```python
from build123d import *

# Parameters (mm, degrees)
SKETCH1_W           = 24.5
SKETCH1_H           = 20.5
BOSS_EXTRUDE1_DEPTH = 4.5
SKETCH2_W           = 0.25
SKETCH2_H           = 0.7
BOSS_EXTRUDE2_DEPTH = 3.5


with BuildPart() as part:
    # Sketch1 → Boss-Extrude1 (new body)
    with BuildSketch(Plane(origin=(0, 0, 0), x_dir=(0, 0, -1), z_dir=(1, 0, 0))):
        Rectangle(SKETCH1_W, SKETCH1_H)
    extrude(amount=BOSS_EXTRUDE1_DEPTH)

    # Sketch2 → Boss-Extrude2 (add)
    with BuildSketch(Plane.XZ.offset(10.25)):
        with Locations((1.2, 7.62)):
            Rectangle(SKETCH2_W, SKETCH2_H)
        with Locations((1.2, 10.16)):
            Rectangle(SKETCH2_W, SKETCH2_H)
        with Locations((1.2, -2.54)):
            Rectangle(SKETCH2_W, SKETCH2_H)
        with Locations((1.2, -10.16)):
            Rectangle(SKETCH2_W, SKETCH2_H)
    extrude(amount=BOSS_EXTRUDE2_DEPTH)


solid = part.part
```
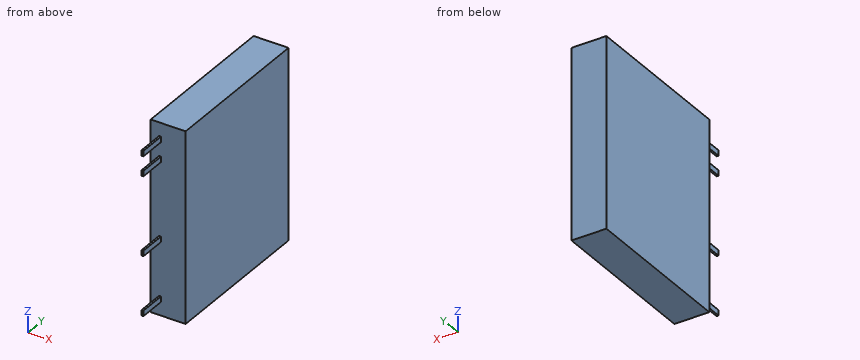
Source: CAD feature listing. Evaluate the final solid. Frame: model axes, mm. Give positions to 0.01 mm unless a question says otherwise; leave off trailing zeros. Write each loop counter-clockwise with the first axis right and the second up, starting at its lowest first coordinate (ties: lowest second). Pieces come first, ordered by that corner, then holes.
1. Section query C-C (z = 4). Return the cut outline in (x, y), then the cut area to 4 significant figures.
2. Material intervals for line 1 along Y through (x, z) = (1.1, -0.25), sorted ascending.
3. Section query B-B (x = 2.2). Return the cut outline in (y, z), then the cut area to 3 significant figures.
4. First-contact query: pin 1 (1 mm diameter, centred on x = 3.5, y = -11, fed in from -Z); pin 2 (1 mm diameter, centred on x = 2, z = 0, fed in from -Y); pin 3 (0.6 mm diameter, centred on y = -11, z = 10, fed in from +X) (3 decimals); pin 4 (0.6 mm diameter, centred on y = -12.5, z = 7.5, fed in from -X) (3 decimals). Flat tips, straight axial feed; report the tip coordinate or a pass-through.
5. Section query A-A (y = -11.5). Return the cut outline in (x, z) (3 decimals).
Output values:
1. outline: (0, -10.25) - (4.5, -10.25) - (4.5, 10.25) - (0, 10.25) - close
1. area: 92.25 mm2
2. line 1: y = -10.25 to 10.25
3. outline: (-10.25, -12.25) - (10.25, -12.25) - (10.25, 12.25) - (-10.25, 12.25) - close
3. area: 502 mm2
4. pin 1: passes through
4. pin 2: stops at y = -10.25
4. pin 3: stops at x = 1.325
4. pin 4: stops at x = 1.075
5. outline: (1.075, -10.51) - (1.325, -10.51) - (1.325, -9.81) - (1.075, -9.81) - close; (1.075, -2.89) - (1.325, -2.89) - (1.325, -2.19) - (1.075, -2.19) - close; (1.075, 7.27) - (1.325, 7.27) - (1.325, 7.97) - (1.075, 7.97) - close; (1.075, 9.81) - (1.325, 9.81) - (1.325, 10.51) - (1.075, 10.51) - close
